Read the model definition and answer for the solid it produces. Units are mm, in the model's axes. A direction names the side the tool comes from. Coordinates: 2 decimals unless noted, no trailing zeros. Loops run counter-clockwise (first coordinate to the right, second up) from the corner with the lowest first, then second, coordinate; pieces in that order, holes last.
Autodesk Inventor part; units mm, degrees
ref_plane "Work Plane1" through (0, 0, 0) normal (0, 0, 1) x (1, 0, 0)
ref_plane "YZ Plane" through (0, 0, 0) normal (1, 0, 0) x (0, 1, 0)
ref_plane "XZ Plane" through (0, 0, 0) normal (0, 1, 0) x (-1, 0, 0)
sketch "Sketch1" plane through (0, 0, 0) normal (0, 0, 1) x (1, 0, 0)
  line L0 (6.35, 70.485) -> (6.35, -70.485)
  line L1 (6.35, -70.485) -> (-6.35, -70.485)
  line L2 (-6.35, -70.485) -> (-6.35, 70.485)
  line L3 (-6.35, 70.485) -> (6.35, -70.485) construction
  line L4 (6.35, 70.485) -> (-6.35, -70.485) construction
  arc A0 (6.2478, 69.3501) -> (-6.2478, 69.3501) centre (0, 70.485) ccw
  circle A1 centre (0, 70.485) radius 2.286
  point P0 (0, 0)
  point P1 (-6.35, 70.485)
  dimension "d0" = 12.7
  dimension "d1" = 140.97
  dimension "d2" = 4.572
extrude "Extrusion1" add sketch "Sketch1" along normal mid plane 12.7
sketch "Sketch2" plane through (6.35, -70.485, 6.35) normal (1, 0, 0) x (0, 0, -1)
  line L0 (3.81, 6.35) -> (8.89, 6.35)
  line L1 (8.89, 6.35) -> (8.89, 126.398)
  line L2 (8.89, 126.398) -> (3.81, 126.398)
  line L3 (3.81, 126.398) -> (3.81, 6.35)
  line L4 (3.81, 6.35) -> (8.89, 126.398) construction
  line L5 (8.89, 6.35) -> (3.81, 126.398) construction
  line L6 (0, 0) -> (12.7, 0)
  line L7 (12.7, 140.97) -> (12.7, 0)
  line L8 (3.81, 126.398) -> (8.89, 126.398)
  line L9 (8.89, 126.398) -> (8.89, 150.398)
  line L10 (8.89, 150.398) -> (3.81, 150.398)
  line L11 (3.81, 150.398) -> (3.81, 126.398)
  point P0 (6.35, 70.485)
  point P1 (6.35, 66.374)
  dimension "d5" = 6.35
  dimension "d6" = 5.08
  dimension "d7" = 3.81
  dimension "d8" = 120.048
  dimension "d9" = 5.08
  dimension "d10" = 24
extrude "Extrusion2" cut sketch "Sketch2" against normal blind 8.89 contours L3 L2 L1 L0
extrude "Extrusion3" cut sketch "Sketch2" against normal through all contours L11 L10 L9 L2
sketch "Sketch3" plane through (0, 0, 6.35) normal (0, 0, 1) x (1, 0, 0)
  circle A0 centre (0, 70.485) radius 2.286
  circle A1 centre (-2.54, 62.531) radius 1.5875
  point P0 (0, 0)
  dimension "d15" = 3.175
  dimension "d16" = 7.954
  dimension "d17" = 2.54
extrude "Extrusion4" cut sketch "Sketch3" against normal through all contours A1
fillet "Fillet1" radius 1.2 14 edges at (-4.445, 55.913, -2.54) (-4.445, 55.913, 2.54) (0, 76.835, 6.35) (-6.35, 0, 6.35) (6.35, 0, 6.35) (0, 76.835, -6.35) (-6.35, 0, -6.35) (6.35, 0, -6.35) (6.35, -70.485, 0) (0, -70.485, 6.35) (-6.35, -70.485, 0) (0, -70.485, -6.35) (1.905, -64.135, -2.54) (1.905, -64.135, 2.54)
sketch "Sketch5" plane through (0, 0, 6.35) normal (0, 0, 1) x (1, 0, 0)
  circle A0 centre (0, 70.485) radius 2.286
  circle A1 centre (0, 70.485) radius 3.302
  point P0 (0, 0)
  dimension "d25" = 6.604
extrude "Extrusion6" cut sketch "Sketch5" against normal blind 1.651
ref_plane "Work Plane1" through (0, 0, 0) normal (0, 0, 1) x (1, 0, 0)
mirror "Mirror1" about plane through (0, 0, 0) normal (0, 0, 1) of "Extrusion6"
sketch "Sketch6" plane through (-6.35, -69.285, 5.15) normal (-1, 0, 0) x (0, 0, 1)
  line L0 (-1.5, 2) -> (-8.5, 2)
  line L1 (-8.5, 2) -> (-8.5, 6)
  line L2 (-8.5, 6) -> (-1.5, 6)
  line L3 (-1.5, 6) -> (-1.5, 2)
  line L4 (-8.5, 16) -> (-1.5, 16)
  line L5 (-8.5, 12) -> (-8.5, 16)
  line L6 (-1.5, 12) -> (-8.5, 12)
  line L7 (-1.5, 16) -> (-1.5, 12)
  line L8 (-8.5, 26) -> (-1.5, 26)
  line L9 (-8.5, 22) -> (-8.5, 26)
  line L10 (-1.5, 22) -> (-8.5, 22)
  line L11 (-1.5, 26) -> (-1.5, 22)
  line L12 (-8.5, 36) -> (-1.5, 36)
  line L13 (-8.5, 32) -> (-8.5, 36)
  line L14 (-1.5, 32) -> (-8.5, 32)
  line L15 (-1.5, 36) -> (-1.5, 32)
  line L16 (0, 0) -> (-10.3, 0)
  line L17 (0, 139.77) -> (0, 0)
  point P0 (-5.15, 69.285)
  dimension "d32" = 7
  dimension "d33" = 4
  dimension "d34" = 10
  dimension "d36" = 2
  dimension "d37" = 1.5
extrude "Extrusion7" cut sketch "Sketch6" against normal blind 10
fillet "Fillet2" radius 0.2 8 edges at (6.35, -63.7835, -2.1885) (6.35, -64.135, 0) (6.35, -63.7835, 2.1885) (6.35, 3.775, 2.54) (-6.35, 56.2645, 2.1885) (-6.35, 55.913, 0) (-6.35, 56.2645, -2.1885) (6.35, 3.775, -2.54)
chamfer "Chamfer1" distance 0.2 angle 45 6 edges at (-3.302, 70.485, 6.35) (-2.286, 70.485, 4.699) (-3.302, 70.485, -6.35) (-2.286, 70.485, -4.699) (-4.1275, 62.531, -6.35) (-4.1275, 62.531, 6.35)
properties part number "Body_Right"
Item 1: Given pin 1 (1 mm diameter, centred on x = 5, z = -3.5, fed in from +Y); pin 2 (2 mm diameter, centred on x = -3.5, z = -0.5, fed in from +Y); pin 3 (2.5 mm diameter, centred on y = -61, z = 0.5, fed in from +X), each flat-ended and moving along its own axis, determine where each tip first touches the part or whether it passes through.
Numbers:
pin 1: stops at y = 74.97
pin 2: stops at y = 55.92
pin 3: stops at x = -2.54
Item 2: A cutting plane is placed at A-A on y = -45. Determine the outline of the cut face in (x, z), then the cut area to 3 significant figures.
Numbers:
outline: (-6.35, -5.15) arc R1.2 ccw to (-5.15, -6.35) - (5.15, -6.35) arc R1.2 ccw to (6.35, -5.15) - (6.35, -2.74) arc R0.2 ccw to (6.15, -2.54) - (3.65, -2.54) - (3.65, -3.35) - (-6.35, -3.35) - close; (-6.35, 3.65) - (3.65, 3.65) - (3.65, 2.54) - (6.15, 2.54) arc R0.2 ccw to (6.35, 2.74) - (6.35, 5.15) arc R1.2 ccw to (5.15, 6.35) - (-5.15, 6.35) arc R1.2 ccw to (-6.35, 5.15) - close
area: 76.3 mm2
Item 3: Determine the mould class of faces 1 (the face through (-0.3, 68.22, 3.51)), 2 (the face through (-4, -53.285, 0)), 3 (the face through (-1, 73, -4.699)) for opening direction Z: released by +Z, released by -Z, zero draft, split by the parting line, or undercut.
Numbers:
face 1: zero draft
face 2: undercut
face 3: released by -Z
Item 4: Find the intervals of material crossed by line 1 along Y through (x, z) = (-4.25, 0.5) (3 decimals); line 2 along Z through (x, y) = (-1.25, 33.5); line 3 along Y through (x, z) = (-5.75, -0.5) (3 decimals), in increasing order.
Numbers:
line 1: y = -70.485 to -67.285, -63.285 to -57.285, -53.285 to -47.285, -43.285 to -37.285, -33.285 to 55.913
line 2: z = -6.35 to -2.54, 2.54 to 6.35
line 3: y = -70.324 to -67.285, -63.285 to -57.285, -53.285 to -47.285, -43.285 to -37.285, -33.285 to 55.913
Item 5: Which of the six approach directions +Z, -Z, +X, -X, +Y, -Y give full straight-line access (tool end or side, diameter ignored) to faces 4 (the face through (-4, -33.285, 0)), 5 (the face through (5, -64.135, 0)), 6 (the face through (1, 8, 2.54))?
Numbers:
face 4: -X
face 5: +X, -X, +Y
face 6: +X, +Y
Item 6: A cutting plane is placed at B-B on y = -23. Determine the outline of the cut face in (x, z), then the cut area to 3 significant figures.
Numbers:
outline: (-6.35, -5.15) arc R1.2 ccw to (-5.15, -6.35) - (5.15, -6.35) arc R1.2 ccw to (6.35, -5.15) - (6.35, -2.74) arc R0.2 ccw to (6.15, -2.54) - (-2.54, -2.54) - (-2.54, 2.54) - (6.15, 2.54) arc R0.2 ccw to (6.35, 2.74) - (6.35, 5.15) arc R1.2 ccw to (5.15, 6.35) - (-5.15, 6.35) arc R1.2 ccw to (-6.35, 5.15) - close
area: 115 mm2
